```python
from build123d import *

# Parameters (mm, degrees)
SKETCH1_W           = 304.8
SKETCH1_H           = 304.8
BOSS_EXTRUDE2_DEPTH = 38.1
FILLET1_R           = 25.4


with BuildPart() as part:
    # Sketch1 → Boss-Extrude2 (new, symmetric)
    with BuildSketch(Plane(origin=(0, 0, 0), x_dir=(1, 0, 0), z_dir=(0, 1, 0))):
        with Locations((152.4, -152.4)):
            Rectangle(SKETCH1_W, SKETCH1_H)
    extrude(amount=BOSS_EXTRUDE2_DEPTH, both=True)

    # Fillet1
    fillet1_edges = [part.edges().sort_by_distance(p)[0] for p in [
        (152.4, 38.1, 304.8),
        (0, 38.1, 152.4),
        (152.4, 38.1, 0),
        (0, 0, 0),
        (0, 0, 304.8),
        (304.8, 0, 304.8),
        (304.8, 0, 0),
        (304.8, 38.1, 152.4),
    ]]
    fillet(fillet1_edges, radius=FILLET1_R)


solid = part.part
```
Verification items for the finished model (mm, model axes). Round coordinates to 2 decimals unless told otherwise and drop trailing zeros. Write each loop counter-clockwise with the first axis right and the second up, starting at its lowest first coordinate (ties: lowest second). Pieces come first, ordered by that corner, then holes. Notation, with made-up numbers: (28, -40) - (83, -40) arc R14 cw to (83, -19) - close; hole circle Ø4 at (61.25, -36). An arc over 180 degrees is marked (long way). Answer as a JSON object with one key per item and string values. Group by question number.
Q1. Go/stop test with flat-tipped pins: pin 1 Ø12 at (x, y) = (165.5, 26.5) entering from -Z; pin 2 Ø3 at (y, z) = (24, 117.5) entering from -X; pin 3 Ø1.5 at (y, z) = (18.5, 93.5) entering from +X. Record where each tip stops, or that it passes through.
Q2. Section check A-A, the plane y = 27.5. Enter the section's corners in (x, z).
Q3. Thickness scan on line 1 (Z direction, x = 256, y = 13); line 2 (Y direction, x = 23.5, z = 41); line 3 (X direction, y = -29, z = 288.5). Record the ranges inside material, lowest first.
Found:
{
 "1": {"pin 1": "stops at z = 1.23", "pin 2": "stops at x = 1.97", "pin 3": "stops at x = 304.29"},
 "2": {"outline": "(4.76, 25.4) arc R20.64 ccw to (25.4, 4.76) - (279.4, 4.76) arc R20.64 ccw to (300.04, 25.4) - (300.04, 279.4) arc R20.64 ccw to (279.4, 300.04) - (25.4, 300.04) arc R20.64 ccw to (4.76, 279.4) - close"},
 "3": {"line 1": "z = 0 to 304.8", "line 2": "y = -38.1 to 38.03", "line 3": "x = 1.69 to 303.11"}
}
